Work out the finished part from the listing and answer in its coordinate system (mm). A direction names the side the tool comes from. Give positions to 0.01 mm unless a question says otherwise; leave off trailing zeros. Loops run counter-clockwise (first coordinate to the right, second up) from the corner with the lowest first, then second, coordinate; pieces in that order, holes last. Notation, with made-up numbers: (-10.75, 0) - (33.25, 0) arc R29 cw to (33.25, 27) - close; hole circle Ø3 at (51.25, 57.25). An arc over 180 degrees is marked (long way). One line per item, written item: value.
from build123d import *

# Parameters (mm, degrees)
BOSS_EXTRUDE1_DEPTH = 0.7
SKETCH2_W           = 3.5
SKETCH2_H           = 3.5
SKETCH2_W_2         = 5.5
SKETCH2_H_2         = 1.5
BOSS_EXTRUDE2_DEPTH = 1.3
SKETCH3_R           = 0.25
BOSS_EXTRUDE3_DEPTH = 3


with BuildPart() as part:
    # Sketch1 → Boss-Extrude1 (new body)
    with BuildSketch(Plane(origin=(0, 0, 0), x_dir=(1, 0, 0), z_dir=(0, 1, 0))):
        Polygon((0, 0), (0, 5), (1.5, 5), (1.5, 8.7), (0.5, 8.7), (0.5, 14.7), (5.5, 14.7), (5.5, 8.7), (4.5, 8.7), (4.5, 5), (6, 5), (6, 0), align=None)
    extrude(amount=BOSS_EXTRUDE1_DEPTH)

    # Sketch2 → Boss-Extrude2 (add)
    with BuildSketch(Plane(origin=(0, 0.7, 0), x_dir=(1, 0, 0), z_dir=(0, 1, 0))):
        with Locations((3, 12.45)):
            Rectangle(SKETCH2_W, SKETCH2_H)
        with Locations((3, 0.75)):
            Rectangle(SKETCH2_W_2, SKETCH2_H_2)
    extrude(amount=BOSS_EXTRUDE2_DEPTH)

    # Sketch3 → Boss-Extrude3 (add)
    with BuildSketch(Plane.XY):
        with Locations(Location((1.095, 1.35, 0), (0, 0, 180))):
            Circle(SKETCH3_R)
        with Locations(Location((2.365, 1.35, 0), (0, 0, 180))):
            Circle(SKETCH3_R)
        with Locations(Location((3.635, 1.35, 0), (0, 0, 180))):
            Circle(SKETCH3_R)
        with Locations(Location((4.905, 1.35, 0), (0, 0, 180))):
            Circle(SKETCH3_R)
    extrude(amount=BOSS_EXTRUDE3_DEPTH)


solid = part.part
1. Section C-C (x = 1.7) is taken. Write down the section's boundary in (y, z).
Output:
outline: (0, -14.7) - (0.7, -14.7) - (0.7, -14.2) - (2, -14.2) - (2, -10.7) - (0.7, -10.7) - (0.7, -1.5) - (2, -1.5) - (2, 0) - (0, 0) - close
2. Find the intervals of material crossed by line 1 along Z through (x, y) = (1.7, 1.3); line 2 along Y through (x, z) = (4.25, -7); line 3 along Z through (x, y) = (5.1, 1.75), in increasing order.
Output:
line 1: z = -14.2 to -10.7, -1.5 to 0
line 2: y = 0 to 0.7
line 3: z = -1.5 to 0
3. Flat-ended cylindrical pins translate along their axes: pin 1 Ø2 at (x, z) = (4, -3.5) entering from +Y; pin 2 Ø0.6 at (y, z) = (0.5, -6) entering from -X; pin 3 Ø0.6 at (x, y) = (4, 0.5) entering from +Z. Find the tip coordinate at first contact, or state that the pin passes through.
Output:
pin 1: stops at y = 0.7
pin 2: stops at x = 1.5
pin 3: stops at z = 0
4. Section A-A (y = 1.35) is taken. Write down the section's boundary in (x, z) (3 decimals), and give its area (3 significant figures).
Output:
outline: (0.25, -1.5) - (5.75, -1.5) - (5.75, 0) - (5.155, 0) - (5.155, 3) - (4.655, 3) - (4.655, 0) - (3.885, 0) - (3.885, 3) - (3.385, 3) - (3.385, 0) - (2.615, 0) - (2.615, 3) - (2.115, 3) - (2.115, 0) - (1.345, 0) - (1.345, 3) - (0.845, 3) - (0.845, 0) - (0.25, 0) - close; (1.25, -14.2) - (4.75, -14.2) - (4.75, -10.7) - (1.25, -10.7) - close
area: 26.5 mm²
5. Section B-B (z = -12.5) is taken. Write down the section's boundary in (x, y).
Output:
outline: (0.5, 0) - (5.5, 0) - (5.5, 0.7) - (4.75, 0.7) - (4.75, 2) - (1.25, 2) - (1.25, 0.7) - (0.5, 0.7) - close
6. Section D-D (x = 2.4) is taken. Write down the section's boundary in (y, z), and give its area (3 significant figures).
Output:
outline: (0, -14.7) - (0.7, -14.7) - (0.7, -14.2) - (2, -14.2) - (2, -10.7) - (0.7, -10.7) - (0.7, -1.5) - (2, -1.5) - (2, 0) - (1.6, 0) - (1.6, 3) - (1.1, 3) - (1.1, 0) - (0, 0) - close
area: 18.3 mm²
7. For faces 1 (the flat face through (3, 1, -10.7)), 2 (the flat face through (0.25, 1, -1)), 3 (the flat face through (3, 1, -14.2)), determine the directions among +Z, -Z, +X, -X, +Y, -Y from which every point of the face is accessible in a straight line to the end or side of a thin tool.
Output:
face 1: +X, -X, +Y
face 2: +Z, -Z, -X, +Y
face 3: -Z, +X, -X, +Y
